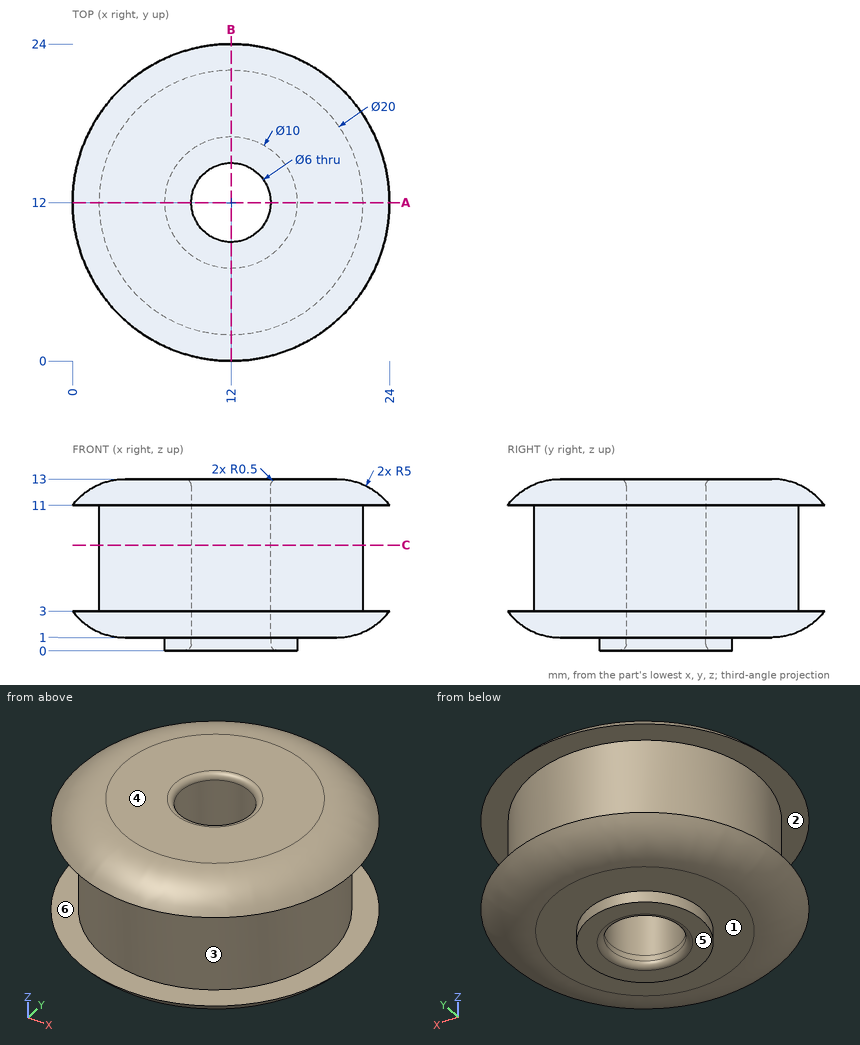
Geometry check sheet. Reference: drawing and pictorial views, mm from the part's lowest x, y, z. A direction names the side the tool comes from. Give positions to 0.01 mm unless a question says otherwise; leave off trailing zeros. Loops run counter-clockwise (first coordinate to the right, second up) from the corner with the lowest first, then second, coordinate; pieces in that order, holes last.
1. Mould release check, pull along Z, two halves, no side actions. Record for the marked faces 1, 2, 3 and 4: released by +Z, released by -Z, zero draft, split by the parting line, or undercut.
2. Section check C-C, the plane z = 8. Enter the section's corners in (x, y), then the cut area to 3 significant figures.
3. Go/stop test with flat-tipped pins: pin 1 Ø12 at (x, y) = (16, 3) entering from -Z; pin 2 Ø2 at (y, z) = (14.5, 5.5) entering from -X; pin 3 Ø1.5 at (x, z) = (21, 11.5) entering from +Y; pin 4 Ø1.5 at (x, z) = (3, 8) entering from +Y. Record where each tip stops, or that it passes through.
4. Thickness scan on line 1 (Y direction, x = 12, z = 9.25); line 2 (Y direction, x = 12, z = 0.7); line 3 (Z direction, x = 14.5, y = 23). Record the ranges inside material, lowest first.
5. Section check A-A, the plane y = 12. Enter the section's corners in (x, z), then the cut area to 3 significant figures.
6. Set-up check for the marked faces 5 and 6: record each of +Z, -Z, +X, -X, +Y, -Y from which the full face is reachable in a straight line by a thin tool's end or side.
Geometry says:
1. face 1: released by -Z
1. face 2: undercut
1. face 3: undercut
1. face 4: released by +Z
2. outline: circle Ø20 at (12, 12); hole circle Ø6 at (12, 12)
2. area: 286 mm2
3. pin 1: stops at z = 0
3. pin 2: stops at x = 2.11
3. pin 3: stops at y = 20.53
3. pin 4: stops at y = 17.65
4. line 1: y = 2 to 9, 15 to 22
4. line 2: y = 7 to 9, 15 to 17
4. line 3: z = 2.23 to 3, 11 to 11.77
5. outline: (0, 3) arc R5 ccw to (4, 1) - (7, 1) - (7, 0) - (8.5, 0) arc R0.5 ccw to (9, 0.5) - (9, 12.5) arc R0.5 ccw to (8.5, 13) - (4, 13) arc R5 ccw to (0, 11) - (2, 11) - (2, 3) - close; (15, 0.5) arc R0.5 ccw to (15.5, 0) - (17, 0) - (17, 1) - (20, 1) arc R5 ccw to (24, 3) - (22, 3) - (22, 11) - (24, 11) arc R5 ccw to (20, 13) - (15.5, 13) arc R0.5 ccw to (15, 12.5) - close
5. area: 178 mm2
6. face 5: -Z, +X, -X, +Y, -Y
6. face 6: none
